Input: part model. Units: mm. Frame: model coordinates. A direction names the side the tool comes from. Coordinates: 2 decimals unless noted, no trailing zeros. Write each loop counter-clockwise with the first axis right and the second up, starting at its lowest first coordinate (ties: lowest second). Pieces come first, ordered by that corner, then holes. Notation, with made-up numbers: (51.25, 84.5) -> (69.25, 84.5) arc R30 cw to (69.25, 110.5) -> close; hole circle Ø6 at (71, -37.5). An arc over 180 degrees is marked (long way). One line per question, with ' | ' between items. Start each with the question number.
```python
from build123d import *

# Parameters (mm, degrees)
F0_W     = 15.24
F0_H     = 15.24
F1_DEPTH = 9
F2_W     = 2
F2_H     = 11.43
F3_DEPTH = 12.7
F4_W     = 4.318
F4_H     = 11.43
F5_DEPTH = 3.6


with BuildPart() as f1:
    # F0 (on Right) → F1 (new body)
    with BuildSketch(Plane.YZ):
        with Locations((-7.62, 7.62)):
            Rectangle(F0_W, F0_H)
    extrude(amount=F1_DEPTH)

    # F2 (on face) → F3 (cut)
    with BuildSketch(Plane(origin=(0, 0, 0), x_dir=(1, 0, 0), z_dir=(0, 0, -1))):
        with Locations((4.5, 7.62)):
            Rectangle(F2_W, F2_H)
    extrude(amount=-F3_DEPTH, mode=Mode.SUBTRACT)

    # F4 (on face) → F5 (cut)
    with BuildSketch(Plane.YZ.offset(9)):
        with Locations((-7.62, 5.715)):
            Rectangle(F4_W, F4_H)
    extrude(amount=-F5_DEPTH, mode=Mode.SUBTRACT)


solid = f1.part
```
1) First-contact query: P1, Ø1.8, axis at x = 7, y = -8.5, coming from the -Z side; P2, Ø3.5, axis at y = -7.5, z = 4, coming from the +X side; P3, Ø1, axis at x = 4.5, y = -5.5, coming from the -Z side. Flat tips, straight axial feed; report the tip coordinate or a pass-through.
2) Section A-A, the plane y = -3. Return loops of the section in (x, z).
3) Pull-direction query (X, two-part tool) for faces 4 (the face through (0, -8, 8)), 5 (the face through (4, -13.335, 6)), 6 (the face through (4, -8, 12.7)), 7 (the face through (4, 0, 8)); classes: released by +X, released by -X, zero draft, split by the parting line, or undercut.
4) Section C-C, the plane x = 3.75. Return loops of the section in (y, z) (3 decimals), then the cut area to 3 significant figures.
5) Section D-D, the plane z = 7.75. Return loops of the section in (x, y) (3 decimals).
6) Ray query, line 1 (Y direction, x = 8, z = 9.75); line 2 (X direction, y = -4, z = 3); line 3 (Z direction, x = 8, y = -7.75). Return the intervals inside material, ascending.
7) Access query for faces 1 (the face through (4, -1.905, 6)), 2 (the face through (9, -4, 8)), 3 (the face through (7, -5.461, 6)). Directions: +Z, -Z, +X, -X, +Y, -Y. A direction counts if a zero-diameter tool reaches every point of the face in a straight line with its end or side. Return the directions, or none.
8) Section B-B, the plane z = 12. Return loops of the section in (x, y) (3 decimals), then the cut area to 3 significant figures.
Answer block:
1) P1: stops at z = 11.43 | P2: stops at x = 3.5 | P3: stops at z = 12.7
2) outline: (0, 0) -> (3.5, 0) -> (3.5, 12.7) -> (5.5, 12.7) -> (5.5, 0) -> (9, 0) -> (9, 15.24) -> (0, 15.24) -> close
3) face 4: released by -X | face 5: undercut | face 6: undercut | face 7: zero draft
4) outline: (-15.24, 0) -> (-13.335, 0) -> (-13.335, 12.7) -> (-1.905, 12.7) -> (-1.905, 0) -> (0, 0) -> (0, 15.24) -> (-15.24, 15.24) -> close | area: 87.1 mm2
5) outline: (0, -15.24) -> (9, -15.24) -> (9, -9.779) -> (5.5, -9.779) -> (5.5, -13.335) -> (3.5, -13.335) -> (3.5, -1.905) -> (5.5, -1.905) -> (5.5, -5.461) -> (9, -5.461) -> (9, 0) -> (0, 0) -> close
6) line 1: y = -15.24 to -9.78, -5.46 to 0 | line 2: x = 0 to 3.5, 5.5 to 9 | line 3: z = 11.43 to 15.24
7) face 1: -Z | face 2: +Z, -Z, +X, +Y, -Y | face 3: -Z, +X
8) outline: (0, -15.24) -> (9, -15.24) -> (9, 0) -> (0, 0) -> close; hole (3.5, -13.335) -> (5.5, -13.335) -> (5.5, -1.905) -> (3.5, -1.905) -> close | area: 114 mm2
